```python
from build123d import *

# Parameters (mm, degrees)
SKETCH1_R           = 36
SKETCH1_R_2         = 20.52
BOSS_EXTRUDE1_DEPTH = 320
CUT_EXTRUDE1_START  = -310
CUT_EXTRUDE1_DEPTH  = 310
BOSS_EXTRUDE2_START = -155
SKETCH3_R           = 20.52
BOSS_EXTRUDE2_DEPTH = 155


with BuildPart() as part:
    # Sketch1 → Boss-Extrude1 (new body)
    with BuildSketch(Plane.XY):
        Polygon((-406.4, -152.64), (406.4, -152.64), (1650.508092605, -152.64), (1650.508092605, 232.64), (-406.4, 232.64), (-406.4, 152.64), align=None)
        Circle(SKETCH1_R, mode=Mode.SUBTRACT)
        with Locations((0, 95.04)):
            Circle(SKETCH1_R_2, mode=Mode.SUBTRACT)
        with Locations((0, -95.04)):
            Circle(SKETCH1_R_2, mode=Mode.SUBTRACT)
    extrude(amount=BOSS_EXTRUDE1_DEPTH)

    # Sketch2 → Cut-Extrude1 (cut)
    with BuildSketch(Plane.XY.offset(320).offset(CUT_EXTRUDE1_START)):
        with BuildLine():
            ThreePointArc((1550, -31), (1571.920310217, -21.920310217), (1581, 0))
            Line((1581, 0), (1581, 186))
            ThreePointArc((1581, 186), (1571.920310217, 207.920310217), (1550, 217))
            Line((1550, 217), (62, 217))
            ThreePointArc((62, 217), (40.079689783, 207.920310217), (31, 186))
            Line((31, 186), (31, 53.469630572))
            Line((31, 53.469630572), (31, 31))
            Line((31, 31), (18.303005218, 31))
            ThreePointArc((18.303005218, 31), (31.264262248, 17.847854383), (36, 0))
            ThreePointArc((36, 0), (31.264262248, -17.847854383), (18.303005218, -31))
            Line((18.303005218, -31), (1550, -31))
        make_face()
    extrude(amount=CUT_EXTRUDE1_DEPTH, mode=Mode.SUBTRACT)

    # Sketch3 → Boss-Extrude2 (add)
    with BuildSketch(Plane.XY.offset(320).offset(BOSS_EXTRUDE2_START)):
        with Locations((0, 95.04)):
            Circle(SKETCH3_R)
        with Locations((0, -95.04)):
            Circle(SKETCH3_R)
    extrude(amount=BOSS_EXTRUDE2_DEPTH)


solid = part.part
```
Could you check a few things on this model? Use its own coordinates, in mm. A direction names the side the tool comes from. Coordinates: 2 decimals unless noted, no trailing zeros. Loops run counter-clockwise (first coordinate to the right, second up) from the corner with the lowest first, then second, coordinate; pieces in that order, holes last.
1) Will this pin go through, and if not, where does the flat tip stop? pin 1 Ø24.5 at (x, y) = (0, -95.04) entering from -Z.
Reported:
pin 1: stops at z = 165
2) Imagine slicing it at A-A (z = 118.5). List the corners of the cut face in (x, y) for me.
Reported:
outline: (-406.4, -152.64) - (1650.51, -152.64) - (1650.51, 232.64) - (-406.4, 232.64) - close; hole circle Ø41.04 at (0, -95.04); hole circle Ø41.04 at (0, 95.04); hole (18.3, -31) - (1550, -31) arc R31 ccw to (1581, 0) - (1581, 186) arc R31 ccw to (1550, 217) - (62, 217) arc R31 ccw to (31, 186) - (31, 31) - (18.3, 31) arc R36 ccw (long way) to start
3) Imagine slicing it at B-B (y = 163.5). List the corners of the cut face in (x, z) for me, and give its area (3 significant figures).
Reported:
outline: (-406.4, 0) - (1650.51, 0) - (1650.51, 320) - (1581, 320) - (1581, 10) - (31, 10) - (31, 320) - (-406.4, 320) - close
area: 178,000 mm2
4) Imagine slicing it at D-D (x = 348). List the corners of the cut face in (y, z) for me, and give its area (3 significant figures).
Reported:
outline: (-152.64, 0) - (232.64, 0) - (232.64, 320) - (217, 320) - (217, 10) - (-31, 10) - (-31, 320) - (-152.64, 320) - close
area: 46,400 mm2
5) Which directions (+Z, -Z, +X, -X, +Y, -Y) give clear straight access to the entire face, cutting with the end or side of a thin tool? Please do faces 5 (the face through (0, -95, 165)), 6 (the face through (1581, 92, 163)), 7 (the face through (608, 43, 0)).
Reported:
face 5: -Z
face 6: +Z
face 7: -Z, +X, -X, +Y, -Y
6) Thinking about a two-plate mould opening in X: for faces 1 (the face through (608, -152.64, 158)), 2 (the face through (1650.508, 37, 158)), 3 (the face through (-4.45, 75.01, 81.34)), 4 (the face through (-406.4, 43, 158)), which applies, released by +X, released by -X, zero draft, split by the parting line, or undercut?
Reported:
face 1: zero draft
face 2: released by +X
face 3: undercut
face 4: released by -X
7) Please list where these lines run through material, in increasing order: line 1 along Y through (x, z) = (0, 43); line 2 along Y through (x, z) = (1287.5, 20); line 3 along X through (y, z) = (111, 216).
Reported:
line 1: y = -152.64 to -115.56, -74.52 to -36, 36 to 74.52, 115.56 to 232.64
line 2: y = -152.64 to -31, 217 to 232.64
line 3: x = -406.4 to 31, 1581 to 1650.51
8) Imagine slicing it at C-C (z = 298). List the corners of the cut face in (x, y) for me, and give its area (3 significant figures).
Reported:
outline: (-406.4, -152.64) - (1650.51, -152.64) - (1650.51, 232.64) - (-406.4, 232.64) - close; hole (18.3, -31) - (1550, -31) arc R31 ccw to (1581, 0) - (1581, 186) arc R31 ccw to (1550, 217) - (62, 217) arc R31 ccw to (31, 186) - (31, 31) - (18.3, 31) arc R36 ccw (long way) to start
area: 405,000 mm2
